Verification items for this drawing (mm, ordinates from the low corner). Give positions to 0.01 mm unless a question says otherwise; leave off trailing zeros. Write each loop counter-clockwise with the first axis right and the second up, starting at its lowest first coordinate (ties: lowest second). Pieces come first, ordered by that corner, then holes. Notation, with made-up numbers: (29.5, 17) -> (54.5, 17) arc R21 cw to (54.5, 54) -> close; hole circle Ø2 at (-6.75, 23.25). An arc over 180 degrees is marked (long way). Write item = value, one per line.
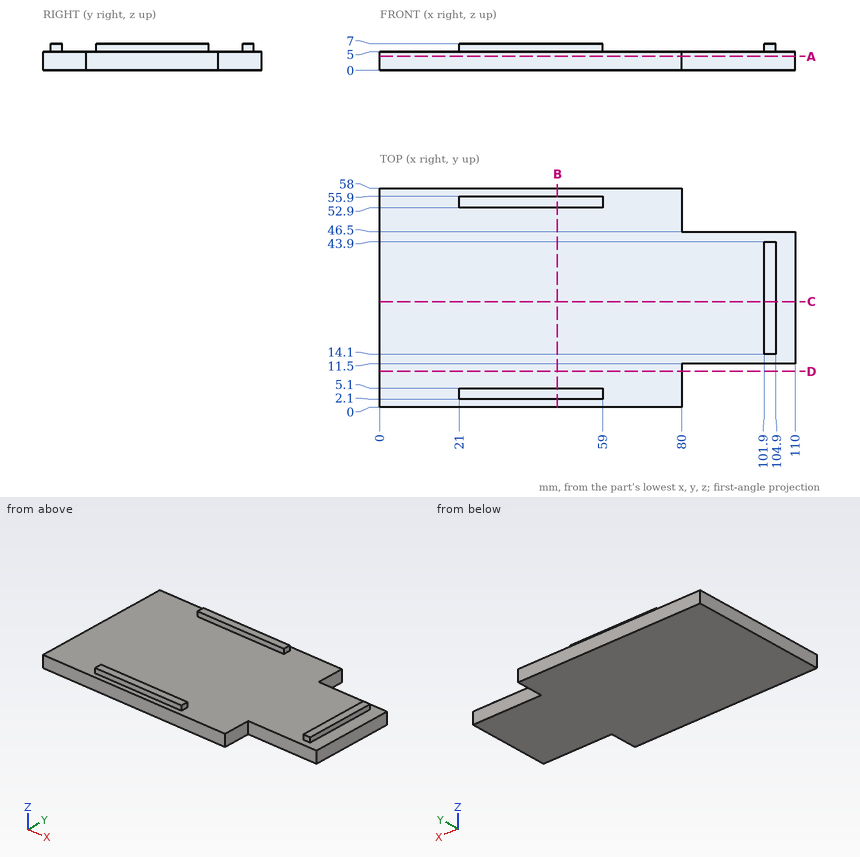
Item 1: Sectioned sample at B-B on x = 47. Record the cut outline in (y, z), then the cut area to 3 significant figures.
Response values:
outline = (0, 0) -> (58, 0) -> (58, 5) -> (55.9, 5) -> (55.9, 7) -> (52.9, 7) -> (52.9, 5) -> (5.1, 5) -> (5.1, 7) -> (2.1, 7) -> (2.1, 5) -> (0, 5) -> close
area = 302 mm^2
Item 2: Material ranges on line 1 (Y direction, x = 46, z = 5.75); line 2 (Y direction, x = 88.5, z = 2); line 3 (Z direction, x = 57.5, y = 14.5), recorded low to high.
Response values:
line_1 = 2.1 to 5.1, 52.9 to 55.9
line_2 = 11.5 to 46.5
line_3 = 0 to 5
Item 3: Sectioned sample at D-D on y = 9.5. Record the cut outline in (x, z), then the cut area to 3 significant figures.
Response values:
outline = (0, 0) -> (80, 0) -> (80, 5) -> (0, 5) -> close
area = 400 mm^2
Item 4: Sectioned sample at A-A on z = 3.75. Record the cut outline in (x, y), then the cut area to 3 significant figures.
Response values:
outline = (0, 0) -> (80, 0) -> (80, 11.5) -> (110, 11.5) -> (110, 46.5) -> (80, 46.5) -> (80, 58) -> (0, 58) -> close
area = 5,690 mm^2
Item 5: Sectioned sample at C-C on y = 28. Record the cut outline in (x, z).
Response values:
outline = (0, 0) -> (110, 0) -> (110, 5) -> (104.9, 5) -> (104.9, 7) -> (101.9, 7) -> (101.9, 5) -> (0, 5) -> close
Item 6: Go/stop test with flat-tipped pins: P1, Ø0.6, axis at y = 53.5, z = 6.5, coming from the +X side; P2, Ø17.5, axis at x = 40.5, y = 25, coming from the +Z side; P3, Ø2, axis at y = 3.5, z = 6.5, coming from the -X side. Record where each tip stops, or that it passes through.
Response values:
P1 = 59
P2 = 5
P3 = 21
